```python
from build123d import *

# Parameters (mm, degrees)
F0_R     = 6.2
F0_R_2   = 5.6
F0_R_3   = 7.5
F1_DEPTH = 1
F2_DEPTH = 11
F3_DEPTH = 11.001
F4_SIZE  = 0.3
F6_DEPTH = 11.001


with BuildPart() as f1:
    # F0 (on Right) → F1 (new body)
    with BuildSketch(Plane.YZ):
        Circle(F0_R)
        Circle(F0_R_2, mode=Mode.SUBTRACT)
        Circle(F0_R_2)
        Circle(F0_R_3)
        Circle(F0_R, mode=Mode.SUBTRACT)
    extrude(amount=F1_DEPTH)

    # F0 (on Right) → F2 (join)
    with BuildSketch(Plane.YZ):
        Circle(F0_R)
        Circle(F0_R_2, mode=Mode.SUBTRACT)
    extrude(amount=F2_DEPTH)

    # F0 (on Right) → F3 (cut, through all)
    with BuildSketch(Plane.YZ):
        Circle(F0_R_2)
    extrude(amount=F3_DEPTH, mode=Mode.SUBTRACT)

    # F4
    f4_edges = [f1.edges().sort_by_distance(p)[0] for p in [
        (0, -5.6, 0),
        (11, -6.2, 0),
        (0, -7.5, 0),
    ]]
    chamfer(f4_edges, length=F4_SIZE)

    # F5 (on Right) → F6 (cut, through all)
    with BuildSketch(Plane.YZ):
        with BuildLine():
            Line((0.588235, 3.956511), (1.25, 8.407586))
            ThreePointArc((1.25, 8.407586), (0, 8.5), (-1.25, 8.407586))
            Line((-1.25, 8.407586), (-0.588235, 3.956511))
            ThreePointArc((-0.588235, 3.956511), (0, 4), (0.588235, 3.956511))
        make_face()
    extrude(amount=F6_DEPTH, mode=Mode.SUBTRACT)


solid = f1.part
```
Could you check a few things on this model? Use its own coordinates, in mm. A direction names the side the tool comes from. Round coordinates to 2 decimals unless told otherwise and drop trailing zeros. Write each loop counter-clockwise with the first axis right and the second up, starting at its lowest first coordinate (ties: lowest second). Pieces come first, ordered by that corner, then holes.
(1) Suppose I cut it at A-A on z = 0. Write out the boundary of the cut face in (x, y).
Findings below:
outline: (0, -7.2) - (0.3, -7.5) - (1, -7.5) - (1, -6.2) - (10.7, -6.2) - (11, -5.9) - (11, -5.6) - (0.3, -5.6) - (0, -5.9) - close; (0, 5.9) - (0.3, 5.6) - (11, 5.6) - (11, 5.9) - (10.7, 6.2) - (1, 6.2) - (1, 7.5) - (0.3, 7.5) - (0, 7.2) - close
(2) Which directions (+Z, -Z, +X, -X, +Y, -Y) give clear straight access to the entire face, cutting with the end or side of a thin tool? Please do faces 5 (the face through (0.115, -0.307, -7.308)), 6 (the face through (5.782, -0.26, -6.195)), 7 (the face through (4.201, -0.872, 5.865)).
Findings below:
face 5: -X
face 6: +X
face 7: +Z, +X, -X
(3) Suppose I cut it at B-B on y = 0. Write out the boundary of the cut face in (x, z), and give its area (4 significant figures).
Findings below:
outline: (0, -7.2) - (0.3, -7.5) - (1, -7.5) - (1, -6.2) - (10.7, -6.2) - (11, -5.9) - (11, -5.6) - (0.3, -5.6) - (0, -5.9) - close
area: 7.765 mm2
(4) If I drill on probe 1 along Y at (x, z) = (8.75, 0); probe 2 along Y at (x, z) = (10.5, -3.5); probe 3 along X at (y, z) = (-2, -6), over which ranges is the centre line in solid material (lowest first)?
Findings below:
probe 1: y = -6.2 to -5.6, 5.6 to 6.2
probe 2: y = -5.12 to -4.37, 4.37 to 5.12
probe 3: x = 0 to 1
(5) Thinking about a two-plate mould opening in Y: for faces 1 (the face through (0, -6, -1)), 2 (the face through (0.645, -0.314, -7.493)), 3 (the face through (5.575, -0.235, -5.595)), 4 (the face through (4.2, 0.87, 5.84)), which applies, +Y half, -Y half, draft (parallel to the pull), parting line (faces both ways), or undercut?
Findings below:
face 1: draft
face 2: parting line
face 3: undercut
face 4: undercut
(6) Suppose I cut it at C-C on x = 9.25. Write out the boundary of the cut face in (y, z), and give its area (3 significant figures).
Findings below:
outline: (-0.91, 6.13) arc R6.2 ccw (long way) to (0.91, 6.13) - (0.82, 5.54) arc R5.6 cw (long way) to (-0.82, 5.54) - close
area: 21.2 mm2
(7) For pin 1 (3 mm diameter, centred on x = 5, z = 4, fed in from -Y); pin 2 (1.5 mm diameter, centred on x = 9, y = 0.5, fed in from -Z); pin 3 (1.5 mm diameter, centred on x = 5.5, y = 4.5, fed in from +Z), each with a flat end and sliding along its axis, tell me the tip position at first contact or that it passes through.
Findings below:
pin 1: stops at y = -5.67
pin 2: stops at z = -6.2
pin 3: stops at z = 4.94
